The model under review builds one solid part; all positions refer to its coordinate system, in mm. Coordinates: 2 decimals unless noted, no trailing zeros. Loops run counter-clockwise (first coordinate to the right, second up) from the corner with the lowest first, then second, coordinate; pieces in that order, holes last. Notation, with made-up numbers: (-23.75, -29) - (9.25, -29) arc R19 cw to (9.25, -15) - close; hole circle Ø6 at (36.25, 84). An arc over 180 degrees is marked (long way). Answer in a Markdown table with one row per item. Add a question column.
(1) We need section C-C on z = 1.8. Give the number of separate pieces and of enclosed holes in the cut face, plus the area to 3 significant figures.
(2) We need section A-A on x = 53.5. Write out the cut boundary in (y, z).
(3) We need section B-B on y = 60.5. Write out the cut boundary in (x, z), plus the area to 3 significant figures.
(4) For P1, Ø1.5, axis at x = 322, z = 1.5, coming from the -Y side; P2, Ø1.5, axis at y = 7, z = 1.5, coming from the -X side; P3, Ø0.9, axis at x = 174.5, z = 2, coming from the -Y side, all flat-tipped, find the tip position at first contact; note any pin that passes through.
(5) For line 1 along X through (y, z) = (6.5, 0.35); line 2 along Y through (x, z) = (161.5, 1.9); line 3 along X through (y, z) = (54, 0.8), list the stretches that pass through material, from the lowest coordinate up.
(6) Mouldability with a two-part tool opening along Y and no side actions: class faces 1 (the cylindrical face through (308.04, 30.7, 1.48)), 2 (the flat face through (159, 35, 3)) as +Y half, -Y half, draft (parallel to the pull), parting line (faces both ways), or undercut.
from build123d import *

# Parameters (mm, degrees)
SKETCH1_R           = 2.5
SKETCH1_W           = 3
SKETCH1_H           = 3
SKETCH1_W_2         = 10
SKETCH1_H_2         = 5
BOSS_EXTRUDE1_DEPTH = 3


with BuildPart() as part:
    # Sketch1 → Boss-Extrude1 (new body)
    with BuildSketch(Plane.XY):
        Polygon((0, 39.585266036), (0, 29.585266036), (3, 29.585266036), (3, 19.585266036), (0, 19.585266036), (0, 9.585266036), (3, 9.585266036), (3, 2.585266036), (64.6, 2.585266036), (64.6, -0.414733964), (129.2, -0.414733964), (129.2, 2.585266036), (193.8, 2.585266036), (193.8, -0.414733964), (258.4, -0.414733964), (258.4, 2.585266036), (320, 2.585266036), (320, 9.585266036), (323, 9.585266036), (323, 19.585266036), (320, 19.585266036), (320, 29.585266036), (323, 29.585266036), (323, 39.585266036), (320, 39.585266036), (320, 66.585266036), (258.4, 66.585266036), (258.4, 69.585266036), (193.8, 69.585266036), (193.8, 66.585266036), (129.2, 66.585266036), (129.2, 69.585266036), (64.6, 69.585266036), (64.6, 66.585266036), (3, 66.585266036), (3, 39.585266036), align=None)
        with Locations((305.733190997, 31.662269088)):
            Circle(SKETCH1_R, mode=Mode.SUBTRACT)
        with Locations((315.5, 7.085266036)):
            Rectangle(SKETCH1_W, SKETCH1_H, mode=Mode.SUBTRACT)
        with Locations((7.5, 7.085266036)):
            Rectangle(SKETCH1_W, SKETCH1_H, mode=Mode.SUBTRACT)
        with Locations((161.5, 22.085266036)):
            Rectangle(SKETCH1_W_2, SKETCH1_H_2, mode=Mode.SUBTRACT)
    extrude(amount=BOSS_EXTRUDE1_DEPTH)


solid = part.part
Outcome:
| question | item | result |
|---|---|---|
| 1 | separate pieces | 1 |
| 1 | enclosed holes | 4 |
| 1 | area | 21,100 mm² |
| 2 | outline | (2.59, 0) - (66.59, 0) - (66.59, 3) - (2.59, 3) - close |
| 3 | outline | (3, 0) - (320, 0) - (320, 3) - (3, 3) - close |
| 3 | area | 951 mm² |
| 4 | P1 | y = 9.59 |
| 4 | P2 | x = 3 |
| 4 | P3 | y = 2.59 |
| 5 | line 1 | 3 to 6, 9 to 314, 317 to 320 |
| 5 | line 2 | 2.59 to 19.59, 24.59 to 66.59 |
| 5 | line 3 | 3 to 320 |
| 6 | face 1 | undercut |
| 6 | face 2 | draft |
